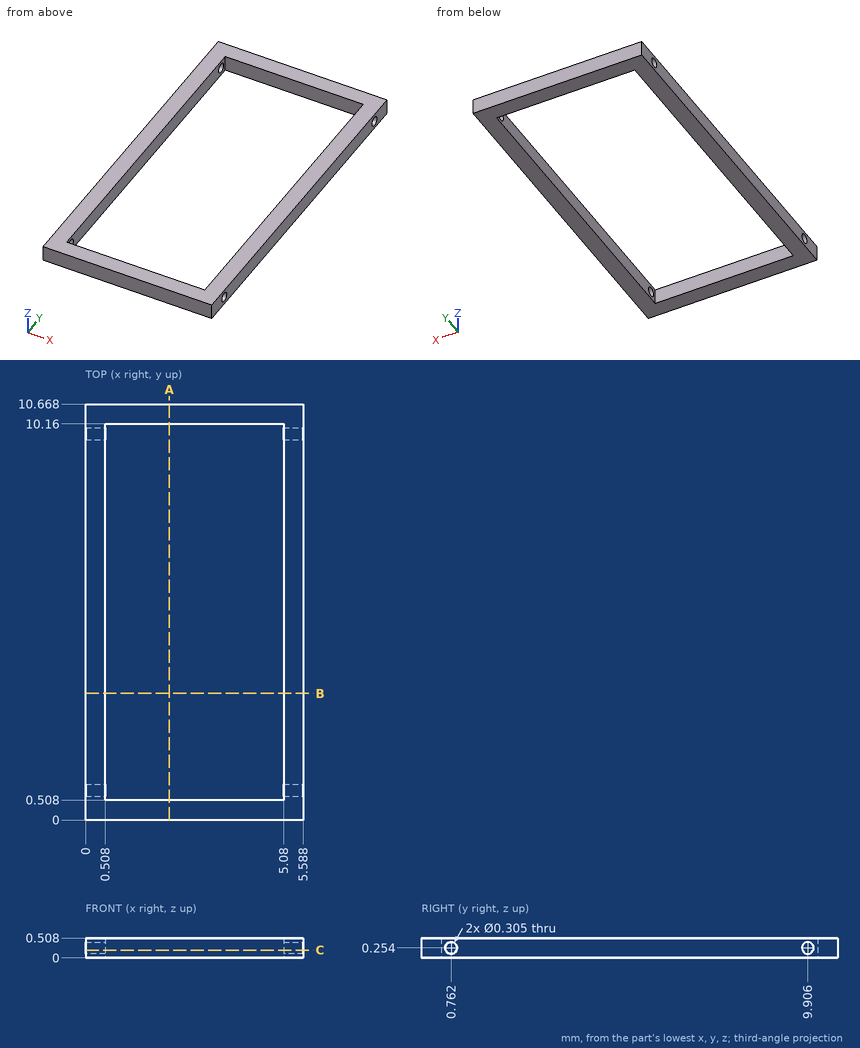
The figure shows three views and two pictorial views of one solid part (mm, origin at its lowest corner). Answer the questions. Round coordinates to 2 decimals unless told otherwise and drop trailing zeros. Write each loop counter-clockwise with the first axis right and the second up, starting at its lowest first coordinate (ties: lowest second). Pieces come first, ordered by that corner, then holes. Notation, with made-up numbers: (-23, 17.5) -> (20, 17.5) arc R22 cw to (20, 45.5) -> close; hole circle Ø1 at (65, -8). An arc over 180 degrees is marked (long way). Answer as a JSON object with one key per item and string values. Group by question number.
Q1. Section A-A (x = 2.15) is taken. Write down the section's boundary in (y, z).
Q2. This flat-tipped pin is pushed along its axis until it touches: pin 1 Ø2 at (x, y) = (2, 9) entering from -Z. Where does it stop, or does it pass through?
Q3. Section B-B (y = 3.25) is taken. Write down the section's boundary in (x, z).
Q4. Section C-C (z = 0.2) is taken. Write down the section's boundary in (x, y).
Q5. Straight lines are drawn through the part: line 1 along Y through (x, z) = (0.4, 0.25); line 2 along X through (y, z) = (10, 0.1); line 3 along Y through (x, z) = (2.3, 0.15). For each, find the intervals that lie inside material, in ascending order.
Check values:
{
 "1": {"outline": "(0, 0) -> (0.51, 0) -> (0.51, 0.51) -> (0, 0.51) -> close; (10.16, 0) -> (10.67, 0) -> (10.67, 0.51) -> (10.16, 0.51) -> close"},
 "2": {"pin 1": "through"},
 "3": {"outline": "(0, 0) -> (0.51, 0) -> (0.51, 0.51) -> (0, 0.51) -> close; (5.08, 0) -> (5.59, 0) -> (5.59, 0.51) -> (5.08, 0.51) -> close"},
 "4": {"outline": "(0, 0) -> (5.59, 0) -> (5.59, 0.62) -> (5.08, 0.62) -> (5.08, 0.51) -> (0.51, 0.51) -> (0.51, 0.62) -> (0, 0.62) -> close; (0, 0.9) -> (0.51, 0.9) -> (0.51, 9.76) -> (0, 9.76) -> close; (0, 10.05) -> (0.51, 10.05) -> (0.51, 10.16) -> (5.08, 10.16) -> (5.08, 10.05) -> (5.59, 10.05) -> (5.59, 10.67) -> (0, 10.67) -> close; (5.08, 0.9) -> (5.59, 0.9) -> (5.59, 9.76) -> (5.08, 9.76) -> close"},
 "5": {"line 1": "0 to 0.61, 0.91 to 9.75, 10.06 to 10.67", "line 2": "0 to 0.51, 5.08 to 5.59", "line 3": "0 to 0.51, 10.16 to 10.67"}
}
